from build123d import *


with BuildPart() as part:
    # Sweep2: sweep along a path in Sketch12
    with BuildLine(Plane(origin=(0, 0, 0), x_dir=(1, 0, 0), z_dir=(0, 1, 0))) as sweep2_path:
        ThreePointArc((0, 0), (-0.074470784, -2.5), (-0.297619048, -4.99113443))
    # Sketch2 → Sweep2 (sweep)
    with BuildSketch(Plane.XY):
        with BuildLine():
            Line((-1.5, -2.8), (1.5, -2.8))
            ThreePointArc((1.5, -2.8), (2.419238816, -2.419238816), (2.8, -1.5))
            Line((2.8, -1.5), (2.8, 1.2))
            add(Edge.make_bspline(
                [(2.8, 1.2), (2.8, 2.022141475), (2.487772802, 2.74054726)],
                knots=[1.570796327, 1.570796327, 1.570796327, 2.078583583, 2.078583583, 2.078583583], degree=2, weights=[1, 0.967941781, 1]))
            ThreePointArc((2.487772802, 2.74054726), (2.288291027, 3.7), (2.487772802, 4.65945274))
            add(Edge.make_bspline(
                [(2.487772802, 4.65945274), (2.8, 5.377858525), (2.8, 6.2)],
                knots=[1.06300907, 1.06300907, 1.06300907, 1.570796327, 1.570796327, 1.570796327], degree=2, weights=[1, 0.967941781, 1]))
            Line((2.8, 6.2), (2.8, 8.9))
            ThreePointArc((2.8, 8.9), (2.419238816, 9.819238816), (1.5, 10.2))
            Line((1.5, 10.2), (-1.5, 10.2))
            ThreePointArc((-1.5, 10.2), (-2.419238816, 9.819238816), (-2.8, 8.9))
            Line((-2.8, 8.9), (-2.8, 6.2))
            add(Edge.make_bspline(
                [(-2.8, 6.2), (-2.8, 5.377858525), (-2.487772802, 4.65945274)],
                knots=[4.71238898, 4.71238898, 4.71238898, 5.220176237, 5.220176237, 5.220176237], degree=2, weights=[1, 0.967941781, 1]))
            ThreePointArc((-2.487772802, 4.65945274), (-2.288291027, 3.7), (-2.487772802, 2.74054726))
            add(Edge.make_bspline(
                [(-2.487772802, 2.74054726), (-2.8, 2.022141475), (-2.8, 1.2)],
                knots=[4.204601724, 4.204601724, 4.204601724, 4.71238898, 4.71238898, 4.71238898], degree=2, weights=[1, 0.967941781, 1]))
            Line((-2.8, 1.2), (-2.8, -1.5))
            ThreePointArc((-2.8, -1.5), (-2.419238816, -2.419238816), (-1.5, -2.8))
        make_face()
        with BuildLine():
            Line((-1.5, -1.5), (1.5, -1.5))
            Line((1.5, -1.5), (1.5, 1.2))
            add(Edge.make_bspline(
                [(1.5, 1.2), (1.5, 3.35), (0, 3.35), (-1.5, 3.35), (-1.5, 1.2)],
                knots=[4.71238898, 4.71238898, 4.71238898, 6.283185307, 6.283185307, 7.853981634, 7.853981634, 7.853981634], degree=2, weights=[1, 0.707106781, 1, 0.707106781, 1]))
            Line((-1.5, 1.2), (-1.5, -1.5))
        make_face(mode=Mode.SUBTRACT)
        with BuildLine():
            Line((1.5, 8.9), (1.5, 6.2))
            add(Edge.make_bspline(
                [(-1.5, 6.2), (-1.5, 4.05), (0, 4.05), (1.5, 4.05), (1.5, 6.2)],
                knots=[4.71238898, 4.71238898, 4.71238898, 6.283185307, 6.283185307, 7.853981634, 7.853981634, 7.853981634], degree=2, weights=[1, 0.707106781, 1, 0.707106781, 1]))
            Line((-1.5, 6.2), (-1.5, 8.9))
            Line((-1.5, 8.9), (1.5, 8.9))
        make_face(mode=Mode.SUBTRACT)
    sweep(path=sweep2_path.line)


solid = part.part
Could you check a few things on this model? Use its own coordinates, in mm. A direction names the side the tool comes from. Give positions to 0.01 mm unless a question says otherwise; leave off trailing zeros. Order: outer loops, then holes, each group sorted by start corner. A loop starts at its lowest first (then second) coordinate and runs counter-clockwise, first axis right, second up.
Item 1: If we mould it in two halves opening along X, with no side actions, what happens to faces 4 (the face through (2.723, -0.131, 2.629)), 5 (the face through (0, 3.8, 0)), 6 (the face through (-1.57, -0.13, 2.38))? For each: pulls with the +X half, pulls with the -X half, needs draft (parallel to the pull), parting line crosses it, or undercut.
Item 2: If we section it at A-A, the plane y = -0.75: Write out the boundary of the cut face in (x, z), plus the area to 3 significant figures.
Item 3: If we section it at B-B, the plane x = -0.15: Count the separate pieces of the cut face and the enclosed holes in it, plus the area to 3 significant figures.
Item 4: For faces 1 (the face through (1.425, -0.169, 2.553)), 2 (the face through (-1.57, 7.57, 2.38)), 3 (the face through (-2.868, 7.531, 2.301)), which set-ups out of +Z, -Z, +X, -X, +Y, -Y let a thin tool reach every point of the face, with its end or its side?
Item 5: If we section it at D-D, the plane y = 9.25: Write out the boundary of the cut face in (x, z), plus the area to 3 significant figures.
Item 6: I'm going to push a flat-ended pin straight in: pin 1 (1 mm diameter, centred on y = 2, z = 2, fed in from +X). Where does the tip first touch, or does it pass through?
Item 7: I need wall thicknesses on line 1 (Y direction, x = -0.2, z = 3.55); line 2 (Y direction, x = 0.9, z = 0.55); line 3 (X direction, y = -0.75, z = 2.4). Which ranges of each line are inside material? Lowest first, please.
Values:
1. face 4: pulls with the +X half
1. face 5: needs draft
1. face 6: undercut
2. outline: (-3.08, 4.66) arc R39.2 cw to (-2.8, 0) - (-1.5, 0) arc R40.5 ccw to (-1.79, 4.81) - close; (1.19, 5.17) arc R43.5 cw to (1.5, 0) - (2.8, 0) arc R44.8 ccw to (2.48, 5.32) - close
2. area: 13.0 mm2
3. separate pieces: 3
3. enclosed holes: 0
3. area: 16.6 mm2
4. face 1: -Z
4. face 2: +Z
4. face 3: -Z, -X, +Y, -Y
5. outline: (-3.03, 4.66) arc R39.25 cw to (-2.75, 0) - (2.75, 0) arc R44.75 ccw to (2.43, 5.32) - close
5. area: 27.5 mm2
6. pin 1: stops at x = 2.75
7. line 1: y = -2.8 to -1.5, 3.35 to 4.05, 8.9 to 10.2
7. line 2: y = -2.8 to -1.5, 2.92 to 4.48, 8.9 to 10.2
7. line 3: x = -2.87 to -1.57, 1.43 to 2.74
